```python
from build123d import *

# Parameters (mm, degrees)
BOSS_EXTRUDE1_DEPTH = 10
FILLET1_R           = 2
SKETCH2_R           = 2.7
CUT_EXTRUDE1_DEPTH  = 41.841155713


with BuildPart() as part:
    # Sketch1 → Boss-Extrude1 (new body)
    with BuildSketch(Plane.XY):
        with BuildLine():
            Line((1, -11.958260743), (1, -14))
            Line((1, -14), (10, -14))
            Line((10, -14), (28, -14))
            Line((28, -14), (28, 14))
            Line((28, 14), (6, 14))
            Line((6, 14), (1, 14))
            Line((1, 14), (1, 11.958260743))
            ThreePointArc((1, 11.958260743), (-2.185898684, 11.799230778), (-5.217338717, 10.806450699))
            Line((-5.217338717, 10.806450699), (-8.841229183, 10.806450699))
            Line((-8.841229183, 10.806450699), (-8.841229183, 8.75))
            Line((-8.841229183, 8.75), (-4.943682838, 8.75))
            ThreePointArc((-4.943682838, 8.75), (10.04990004, 0.04482392), (-4.865435329, -8.79375))
            Line((-4.865435329, -8.79375), (-8.841229183, -8.79375))
            Line((-8.841229183, -8.79375), (-8.841229183, -10.849241119))
            Line((-8.841229183, -10.849241119), (-5.127764341, -10.849241119))
            ThreePointArc((-5.127764341, -10.849241119), (-2.137075278, -11.808171292), (1, -11.958260743))
        make_face()
    extrude(amount=BOSS_EXTRUDE1_DEPTH)

    # Fillet1
    fillet1_edges = [part.edges().sort_by_distance(p)[0] for p in [
        (28, 0, 0),
        (-8.841229183, 8.75, 5),
        (-5.217338717, 10.806450699, 5),
        (1, 11.958260743, 5),
        (1, -11.958260743, 5),
        (-5.127764341, -10.849241119, 5),
        (-8.841229183, -8.79375, 5),
        (28, 0, 10),
    ]]
    fillet(fillet1_edges, radius=FILLET1_R)

    # Sketch2 → Cut-Extrude1 (cut, through all)
    with BuildSketch(Plane.XZ.offset(14)):
        with Locations(Location((13, 5, 0), (0, 0, 270))):
            Circle(SKETCH2_R)
        with Locations(Location((22, 5, 0), (0, 0, 270))):
            Circle(SKETCH2_R)
    extrude(amount=-CUT_EXTRUDE1_DEPTH, mode=Mode.SUBTRACT)


solid = part.part
```
Model file for the job. Use its own axes, mm. A direction names the side the tool comes from. Coordinates: 2 decimals unless noted, no trailing zeros. Write each loop counter-clockwise with the first axis right and the second up, starting at its lowest first coordinate (ties: lowest second). Pieces come first, ordered by that corner, then holes. Notation, with made-up numbers: (9, 86.5) - (16, 86.5) arc R18 cw to (16, 95.5) - close; hole circle Ø1 at (83.5, 41.25). An arc over 180 degrees is marked (long way). One line per item, written item: value. Start each with the question number.
1. Tool access for faces 1 (the flat face through (-7, -10.849, 5)), 2 (the flat face through (-6, -8.794, 5)), 3 (the flat face through (-7, 10.806, 5)): list every direction of +Z, -Z, +X, -X, +Y, -Y with a clear straight run to the whole face (end or side of a thin tool).
2. Flat gauge pins, fed straight in: pin 1 (1.6 mm diameter, centred on x = -8, z = 7.5, fed in from +Y); pin 2 (3 mm diameter, centred on y = 7, z = 8, fed in from -X); pin 3 (1.5 mm diameter, centred on x = -5.5, z = 7, fed in from -Y). Where does each tip first touch, or does it go through?
3. Slice it at C-C (y = 0). Write the cut outline in (x, z).
4. Slice it at B-B (x = 13). Write the cut outline in (y, z).
5. Slice it at D-D (x = 5.5). Write the cut outline in (y, z), plus the area to 3 significant figures.
6. Mould opens along Z. For faces 4 (the cylindrical face through (27.43, 0.2, 9.4)), 5 (the cylindrical face through (27.43, 0.2, 0.6)), 6 (the cylindrical face through (-5.24, 10.85, 5.07)), 7 (the cylindrical face through (24.677, -0.196, 5.351)) say: released by +Z, released by -Z, zero draft, split by the parting line, or undercut.
7. Probe line 1 (Y direction, x = -5.5, z = 9.25); line 2 (X direction, y = 5, z = 5); line 3 (X direction, y = -8, z = 5). List the from-to ranges inside material, lowest first. Write a range as from..to.
8. Slice it at A-A (z = 5). Count the separate pieces of the cut face and the enclosed holes in it, plus the area to 3 significant figures.
Answers below:
1. face 1: +Z, -Z, -X, -Y
1. face 2: +Z, -Z, -X
1. face 3: +Z, -Z, -X, +Y
2. pin 1: stops at y = 10.81
2. pin 2: stops at x = 5.36
2. pin 3: stops at y = -11.02
3. outline: (10.05, 0) - (26, 0) arc R2 ccw to (28, 2) - (28, 8) arc R2 ccw to (26, 10) - (10.05, 10) - close; hole circle Ø5.4 at (13, 5); hole circle Ø5.4 at (22, 5)
4. outline: (-14, 0) - (14, 0) - (14, 2.3) - (-14, 2.3) - close; (-14, 7.7) - (14, 7.7) - (14, 10) - (-14, 10) - close
5. outline: (-14, 0) - (-8.41, 0) - (-8.41, 10) - (-14, 10) - close; (8.41, 0) - (14, 0) - (14, 10) - (8.41, 10) - close
5. area: 112 mm^2
6. face 4: released by +Z
6. face 5: released by -Z
6. face 6: zero draft
6. face 7: undercut
7. line 1: y = -10.85..-8.79, 8.75..10.81
7. line 2: x = 8.72..10.3, 15.7..19.3, 24.7..28
7. line 3: x = 6.08..10.3, 15.7..19.3, 24.7..28
8. separate pieces: 3
8. enclosed holes: 0
8. area: 355 mm^2
